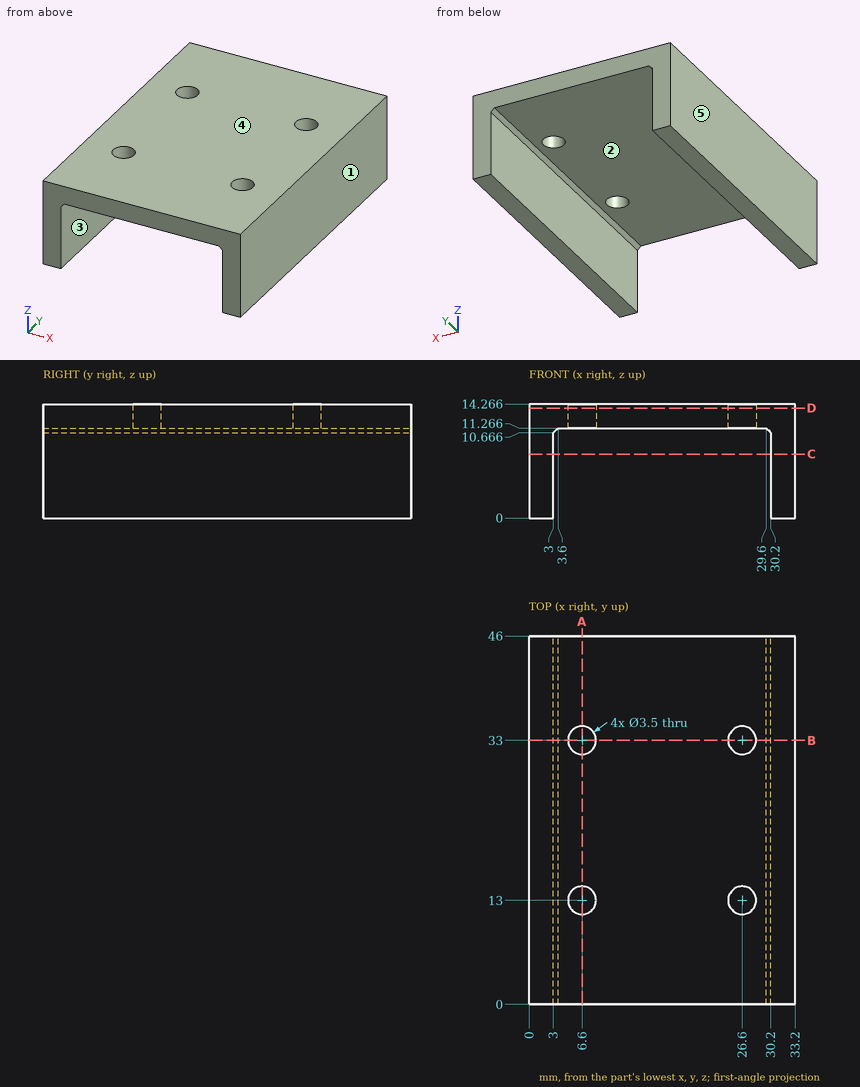
The figure shows three views and two pictorial views of one solid part (mm, origin at its lowest corner). Answer the questions. A direction names the side the tool comes from. Coordinates: 2 decimals unless noted, no trailing zeros. Loops run counter-clockwise (first coordinate to the right, second up) from the corner with the lowest first, then second, coordinate; pieces in that order, holes last.
1) Find section C-C on z = 8. Write down the section's boundary in (x, y).
2) Flat-ended cylindrical pins translate along their axes: pin 1 Ø2 at (x, y) = (26.6, 13) entering from -Z; pin 2 Ø5 at (x, y) = (27.5, 40) entering from -Z; pin 3 Ø13 at (x, y) = (22.5, 31.5) entering from -Z. Find the tip coordinate at first contact, or state that the pin passes through.
3) Find section D-D on z = 13.75. Write down the section's boundary in (x, y), then the cut area to 3 significant figures.
4) Find section B-B on y = 33. Write down the section's boundary in (x, z).
5) Determine the mould class of the marked faces 3, 4 and 5 for opening direction X: pulls with the +X half, pulls with the -X half, needs draft (parallel to the pull), parting line crosses it, or undercut.
6) Find the intervals of material crossed by L1, parallel to Y at x = 6.6, z = 13; L2, parallel to X at y = 11, z = 8.75; L3, parallel to X at y = 33.5, z = 13.25, in increasing order.
7) Find section A-A on x = 6.6. Write down the section's boundary in (y, z).
8) A tool of negligible diameter and unlimited length cuts with its end or side. For the marked faces 1 and 2, from which of +Z, -Z, +X, -X, +Y, -Y can it reach the whole face along a straight path? Write none if from no direction.
Values:
1. outline: (0, 0) - (3, 0) - (3, 46) - (0, 46) - close; (30.2, 0) - (33.2, 0) - (33.2, 46) - (30.2, 46) - close
2. pin 1: passes through
2. pin 2: stops at z = 10.87
2. pin 3: stops at z = 11.27
3. outline: (0, 0) - (33.2, 0) - (33.2, 46) - (0, 46) - close; hole circle Ø3.5 at (6.6, 13); hole circle Ø3.5 at (6.6, 33); hole circle Ø3.5 at (26.6, 13); hole circle Ø3.5 at (26.6, 33)
3. area: 1,490 mm2
4. outline: (0, 0) - (3, 0) - (3, 10.67) - (3.6, 11.27) - (4.85, 11.27) - (4.85, 14.27) - (0, 14.27) - close; (8.35, 11.27) - (24.85, 11.27) - (24.85, 14.27) - (8.35, 14.27) - close; (28.35, 11.27) - (29.6, 11.27) - (30.2, 10.67) - (30.2, 0) - (33.2, 0) - (33.2, 14.27) - (28.35, 14.27) - close
5. face 3: undercut
5. face 4: needs draft
5. face 5: pulls with the -X half
6. L1: y = 0 to 11.25, 14.75 to 31.25, 34.75 to 46
6. L2: x = 0 to 3, 30.2 to 33.2
6. L3: x = 0 to 4.92, 8.28 to 24.92, 28.28 to 33.2
7. outline: (0, 11.27) - (11.25, 11.27) - (11.25, 14.27) - (0, 14.27) - close; (14.75, 11.27) - (31.25, 11.27) - (31.25, 14.27) - (14.75, 14.27) - close; (34.75, 11.27) - (46, 11.27) - (46, 14.27) - (34.75, 14.27) - close
8. face 1: +Z, -Z, +X, +Y, -Y
8. face 2: -Z, +Y, -Y
